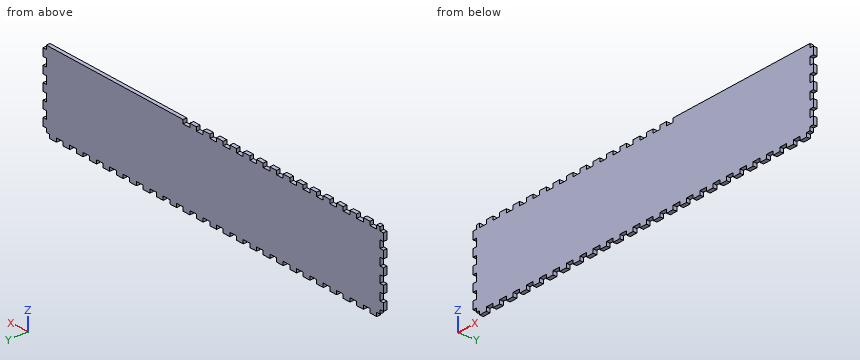
```python
from build123d import *

# Parameters (mm, degrees)
SKETCH003_W             = 500
SKETCH003_H             = 100
PAD003_DEPTH            = 5
SKETCH025_W             = 10
SKETCH025_H             = 5
PAD023_DEPTH            = 5
LINEARPATTERN005_COUNT  = 25
LINEARPATTERN005_PITCH  = 20
SKETCH026_W             = 10
SKETCH026_H             = 5
PAD024_DEPTH            = 5
LINEARPATTERN006_COUNT  = 5
LINEARPATTERN006_PITCH  = 20
SKETCH027_W             = 10
SKETCH027_H             = 5
PAD025_DEPTH            = 5
LINEARPATTERN007_COUNT  = 5
LINEARPATTERN007_PITCH  = 20
SKETCH122_W             = 10
SKETCH122_H             = 5
POCKET032_DEPTH         = 5
LINEARPATTERN074_COUNT  = 15
LINEARPATTERN074_PITCH  = 20
BODY003_PLACEMENT_ANGLE = 90


with BuildPart() as part:
    # Sketch003 → Pad003 (new body)
    with BuildSketch(Plane.XY):
        Rectangle(SKETCH003_W, SKETCH003_H)
    extrude(amount=PAD003_DEPTH)

    # Sketch025 (on DatumPlane) → Pad023 (join)
    with BuildSketch(Plane.XZ.offset(50)):
        with Locations((-240, 2.5)):
            Rectangle(SKETCH025_W, SKETCH025_H)
    pad023 = extrude(amount=PAD023_DEPTH)

    # LinearPattern005: Pad023 ×25
    with Locations(*[(i * LINEARPATTERN005_PITCH, 0, 0) for i in range(1, LINEARPATTERN005_COUNT)]):
        add(pad023)

    # Sketch026 (on DatumPlane) → Pad024 (join)
    with BuildSketch(Plane.YZ.offset(250)):
        with Locations((-40, 2.5)):
            Rectangle(SKETCH026_W, SKETCH026_H)
    pad024 = extrude(amount=PAD024_DEPTH)

    # LinearPattern006: Pad024 ×5
    with Locations(*[(0, i * LINEARPATTERN006_PITCH, 0) for i in range(1, LINEARPATTERN006_COUNT)]):
        add(pad024)

    # Sketch027 (on DatumPlane) → Pad025 (join)
    with BuildSketch(Plane(origin=(-250, 0, 0), x_dir=(0, -1, 0), z_dir=(-1, 0, 0))):
        with Locations((-40, 2.5)):
            Rectangle(SKETCH027_W, SKETCH027_H)
    pad025 = extrude(amount=PAD025_DEPTH)

    # LinearPattern007: Pad025 ×5
    with Locations(*[(0, -i * LINEARPATTERN007_PITCH, 0) for i in range(1, LINEARPATTERN007_COUNT)]):
        add(pad025)

    # Sketch122 (on DatumPlane) → Pocket032 (cut)
    with BuildSketch(Plane(origin=(0, 50, 0), x_dir=(-1, 0, 0), z_dir=(0, 1, 0))):
        with Locations((240, 2.5)):
            Rectangle(SKETCH122_W, SKETCH122_H)
    pocket032 = extrude(amount=-POCKET032_DEPTH, mode=Mode.SUBTRACT)

    # LinearPattern074: Pocket032 ×15
    with Locations(*[(i * LINEARPATTERN074_PITCH, 0, 0) for i in range(1, LINEARPATTERN074_COUNT)]):
        add(pocket032, mode=Mode.SUBTRACT)


with BuildPart() as part_1:
    # Body003 placement: moved
    add(part.part.moved(Location((0, -145, 55))).rotate(Axis((0, -145, 55), (1, 0, 0)), BODY003_PLACEMENT_ANGLE))


solid = part_1.part
```
Part model, mm, in its own coordinate system. Coordinates: 2 decimals unless noted, no trailing zeros. Order: outer loops, then holes, each group sorted by start corner. A loop starts at its lowest first (then second) coordinate and runs counter-clockwise, first axis right, second up. Notation, with made-up numbers: (21, 63.5) -> (67, 63.5) arc R8 cw to (67, 75.5) -> close; hole circle Ø8 at (23, -38). An arc over 180 degrees is marked (long way). Put each result on its own line as item: value. Start each with the question number.
(1) Pin check, flat tips, straight feed: pin 1 Ø2.5 at (x, y) = (188, -147.5) entering from -Z; pin 2 Ø2.5 at (x, y) = (252.5, -148.5) entering from +Z; pin 3 Ø1.5 at (y, z) = (-148, 1.5) entering from +X. Stop position of each tip, or through.
(2) Probe line 1 along X through (y, z) = (-149.15, 87.5); line 2 along Z through (x, y) = (-67, -148.6); line 3 along Z through (x, y) = (-62.5, -145.3). List the from-to ranges inside material, lowest first. Write a range as [from, to].
(3) Band-saw the part on A-A (x = -10.5). Give the cut face in (y, z), then the cut area to 3 significant figures.
Determined:
1. pin 1: stops at z = 5
1. pin 2: stops at z = 100
1. pin 3: stops at x = 245
2. line 1: x = [-250, 250]
2. line 2: z = [5, 105]
2. line 3: z = [0, 100]
3. outline: (-150, 5) -> (-145, 5) -> (-145, 105) -> (-150, 105) -> close
3. area: 500 mm²
